Check sheet for the modelled part. Datum: model origin and axes. Units: mm. Face numbers are marked on the shaded views. A direction names the side the tool comes from. Coordinates: 2 decimals unless noted, no trailing zeros. Write each loop counter-clockwise with the first axis right and the second up, starting at its lowest first coordinate (ties: lowest second). Pieces come first, ordered by that corner, then holes. Notation, with made-up numbers: M 63,68 L 111,68 A10 cw 111,75 Z; hole C 22.25,-21 d9. An arc over 180 degrees is marked long. Answer as CSV lines item,"result". Start each with the question number.
1) Access from +Z, -Z, +X, -X, +Y, -Y to the whole of each face (thin tool, end or side, straight path). Record for the marked faces 4 and 5.
2) Section check D-D (x = 0). State how many separate pieces and enclosed holes the cut face has, and give its area (3 significant figures).
3) Draft check along X on the marked faces 1, 2 and 3. Enter one of: +X half, -X half, draft (parallel to the pull), parting line (faces both ways), or undercut.
4) Material ranges on L1, parallel to Z at x = -42.5, y = 4.75; L2, parallel to Z at x = -39, y = -5; L3, parallel to X at y = -4.5, z = -26, recorded low to high. Write a range as [from, to].
5) Section check A-A (z = 0). Record the cut outline in (x, y), and give its area (3 significant figures).
6) Section check C-C (z = 24.5). Record the cut outline in (x, y).
7) Go/stop test with flat-tipped pins: pin 1 Ø17.5 at (x, z) = (2, -1) entering from +Y; pin 2 Ø9.5 at (x, z) = (0, -49) entering from +Y; pin 3 Ø8 at (x, y) = (-29.5, -4.5) entering from +Z; pin 4 Ø7 at (x, z) = (42.44, 24.5) entering from -Y. Record where each tip stops, or that it passes through.
8) Section check B-B (y = -4.5). Record the cut outline in (x, z).
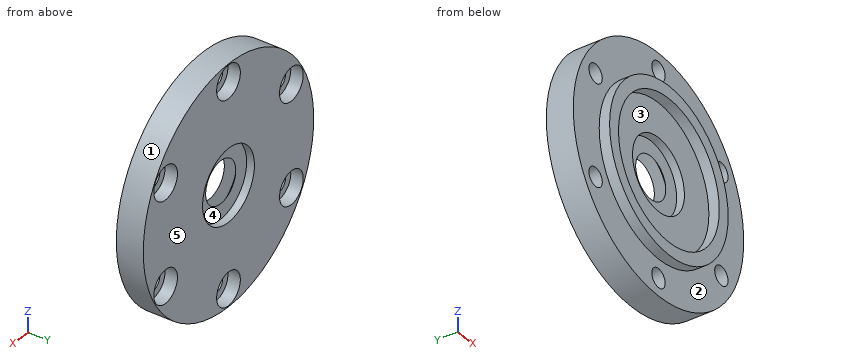
from build123d import *

# Parameters (mm, degrees)
SKETCH_1_R               = 57.5
EXTRUDE_1_DEPTH          = 6.5
SKETCH_3_R               = 8
CUT_EXTRUDE_1_DEPTH      = 6
SKETCH_4_R               = 4.5
CUT_EXTRUDE_2_DEPTH      = 82.618012718
PATTERN_CIRCULAR_1_COUNT = 6
SKETCH_6_R               = 17.5
CUT_EXTRUDE_3_DEPTH      = 3.75
SKETCH_9_R               = 17.5
CUT_EXTRUDE_4_DEPTH      = 3.75
SKETCH_10_R              = 40
SKETCH_10_R_2            = 34
EXTRUDE_2_DEPTH          = 5


with BuildPart() as part:
    # 草图1 → 凸台-拉伸1 (new, symmetric)
    with BuildSketch(Plane(origin=(0, 0, 0), x_dir=(1, 0, 0), z_dir=(0, 1, 0))):
        with Locations(Location((0, 0, 0), (0, 0, 90))):
            Circle(SKETCH_1_R)
    extrude(amount=EXTRUDE_1_DEPTH, both=True)

    # 草图3 → 切除-拉伸1 (cut)
    with BuildSketch(Plane(origin=(0, 6.5, 0), x_dir=(1, 0, 0), z_dir=(0, 1, 0))):
        with Locations(Location((0, 49, 0), (0, 0, 270))):
            Circle(SKETCH_3_R)
    cut_extrude_1 = extrude(amount=-CUT_EXTRUDE_1_DEPTH, mode=Mode.SUBTRACT)

    # 草图4 → 切除-拉伸2 (cut, through all)
    with BuildSketch(Plane(origin=(0, 0.5, 0), x_dir=(1, 0, 0), z_dir=(0, 1, 0))):
        with Locations(Location((0, 49, 0), (0, 0, 270))):
            Circle(SKETCH_4_R)
    cut_extrude_2 = extrude(amount=-CUT_EXTRUDE_2_DEPTH, mode=Mode.SUBTRACT)

    # 阵列(圆周)1: 切除-拉伸1, 切除-拉伸2 ×6 about axis
    pattern_circular_1_axis = Axis((0, 0, 0), (0, 1, 0))
    add([cut_extrude_1.rotate(pattern_circular_1_axis, i * 360 / PATTERN_CIRCULAR_1_COUNT) for i in range(1, PATTERN_CIRCULAR_1_COUNT)], mode=Mode.SUBTRACT)
    add([cut_extrude_2.rotate(pattern_circular_1_axis, i * 360 / PATTERN_CIRCULAR_1_COUNT) for i in range(1, PATTERN_CIRCULAR_1_COUNT)], mode=Mode.SUBTRACT)

    # 草图6 → 切除-拉伸3 (cut)
    with BuildSketch(Plane(origin=(0, 6.5, 0), x_dir=(1, 0, 0), z_dir=(0, 1, 0))):
        with Locations(Location((0, 0, 0), (0, 0, 270))):
            Circle(SKETCH_6_R)
    extrude(amount=-CUT_EXTRUDE_3_DEPTH, mode=Mode.SUBTRACT)

    # 草图8 → 切除-旋转1 (revolve, cut)
    with BuildSketch(Plane.XY, mode=Mode.PRIVATE) as cut_revolve_1_sk:
        Polygon((-10.158018271, 2.75), (-18.189384238, 2), (-18.189384238, -2), (-10.158018271, -2.75), (0, -2.75), (0, 2.75), align=None)
    revolve(cut_revolve_1_sk.sketch.rotate(Axis((0, 37.664252475, 0), (0, -1, 0)), 270), axis=Axis((0, 37.664252475, 0), (0, -1, 0)), mode=Mode.SUBTRACT)

    # 草图9 → 切除-拉伸4 (cut)
    with BuildSketch(Plane(origin=(0, -2.75, 0), x_dir=(1, 0, 0), z_dir=(0, 1, 0))):
        with Locations(Location((0, 0, 0), (0, 0, 270))):
            Circle(SKETCH_9_R)
    extrude(amount=-CUT_EXTRUDE_4_DEPTH, mode=Mode.SUBTRACT)

    # 草图10 → 凸台-拉伸2 (add)
    with BuildSketch(Plane.XZ.offset(6.5)):
        with Locations(Location((0, 0, 0), (0, 0, 90))):
            Circle(SKETCH_10_R)
        with Locations(Location((0, 0, 0), (0, 0, 270))):
            Circle(SKETCH_10_R_2, mode=Mode.SUBTRACT)
    extrude(amount=EXTRUDE_2_DEPTH)


solid = part.part
Results found:
1,face 4,"+Y"
1,face 5,"+Z, -Z, +X, -X, +Y"
2,separate pieces,"4"
2,enclosed holes,"0"
2,area,"786 mm2"
3,face 1,"parting line"
3,face 2,"draft"
3,face 3,"undercut"
4,L1,"z = [-38.73, -32.5], [-16.5, 16.5], [32.5, 38.73]"
4,L2,"z = [-42.25, -27.41], [-21.59, 21.59], [27.41, 42.25]"
4,L3,"x = [-51.29, -46.68], [-38.19, 38.19], [46.68, 51.29]"
5,outline,"M -57.5,-6.5 L -40,-6.5 L -40,-11.5 L -34,-11.5 L -34,-6.5 L -17.5,-6.5 L -17.5,-2.75 L -10.16,-2.75 L -18.19,-2 L -18.19,2 L -10.16,2.75 L -17.5,2.75 L -17.5,6.5 L -57.5,6.5 Z; M 10.16,-2.75 L 17.5,-2.75 L 17.5,-6.5 L 34,-6.5 L 34,-11.5 L 40,-11.5 L 40,-6.5 L 57.5,-6.5 L 57.5,6.5 L 17.5,6.5 L 17.5,2.75 L 10.16,2.75 L 18.19,2 L 18.19,-2 Z"
5,area,"1,100 mm2"
6,outline,"M -52.02,-6.5 L -46.94,-6.5 L -46.94,0.5 L -50.44,0.5 L -50.44,6.5 L -52.02,6.5 Z; M -37.94,-6.5 L -31.62,-6.5 L -31.62,-11.5 L -23.57,-11.5 L -23.57,-6.5 L 23.57,-6.5 L 23.57,-11.5 L 31.62,-11.5 L 31.62,-6.5 L 37.94,-6.5 L 37.94,0.5 L 34.44,0.5 L 34.44,6.5 L -34.44,6.5 L -34.44,0.5 L -37.94,0.5 Z; M 46.94,-6.5 L 52.02,-6.5 L 52.02,6.5 L 50.44,6.5 L 50.44,0.5 L 46.94,0.5 Z"
7,pin 1,"stops at y = 2.75"
7,pin 2,"stops at y = 0.5"
7,pin 3,"stops at z = 51.54"
7,pin 4,"passes through"
8,outline,"C 0,0 d115; hole C -42.44,-24.5 d9; hole C -42.44,24.5 d9; hole C 0,0 d35; hole C 0,-49 d9; hole C 0,49 d9; hole C 42.44,-24.5 d9; hole C 42.44,24.5 d9"
